Read the model definition and answer for the solid it produces. Units are mm, in the model's axes. A direction names the side the tool comes from. Coordinates: 2 decimals unless noted, no trailing zeros. Loops run counter-clockwise (first coordinate to the right, second up) from the corner with the lowest first, then second, coordinate; pieces in that order, holes last. Notation, with made-up numbers: (12.5, 65.5) - (49.5, 65.5) arc R30 cw to (49.5, 101.5) - close; hole circle Ø5 at (22, 7.25). An arc over 180 degrees is marked (long way). Use CSV: the item, a comma, the result in double quotes.
```python
from build123d import *

# Parameters (mm, degrees)
BOSS_EXTRUDE5_DEPTH = 3.175
SKETCH8_R           = 1.27
BOSS_EXTRUDE6_DEPTH = 3.302
CUT_EXTRUDE3_DEPTH  = 30.47138916


with BuildPart() as part:
    # Sketch7 → Boss-Extrude5 (new body)
    with BuildSketch(Plane(origin=(0, 0, 0), x_dir=(1, 0, 0), z_dir=(0, 1, 0))):
        with BuildLine():
            Line((-3.175, 25.4), (-3.175, -25.4))
            ThreePointArc((-3.175, -25.4), (0, -28.575), (3.175, -25.4))
            Line((3.175, -25.4), (3.175, 25.4))
            ThreePointArc((3.175, 25.4), (0, 28.575), (-3.175, 25.4))
        make_face()
    extrude(amount=BOSS_EXTRUDE5_DEPTH)

    # Sketch8 → Boss-Extrude6 (add)
    with BuildSketch(Plane(origin=(0, 3.175, 0), x_dir=(1, 0, 0), z_dir=(0, 1, 0))):
        with Locations(Location((0, 25.4, 0), (0, 0, 90))):
            Circle(SKETCH8_R)
        with Locations(Location((0, -25.4, 0), (0, 0, 90))):
            Circle(SKETCH8_R)
    extrude(amount=BOSS_EXTRUDE6_DEPTH)

    # Sketch9 → Cut-Extrude3 (cut, through all)
    with BuildSketch(Plane.XZ):
        with BuildLine():
            Line((-1.866511184, 1.905), (-1.866511184, -1.905))
            ThreePointArc((-1.866511184, -1.905), (0, -2.667), (1.866511184, -1.905))
            Line((1.866511184, -1.905), (1.866511184, 1.905))
            ThreePointArc((1.866511184, 1.905), (0, 2.667), (-1.866511184, 1.905))
        make_face()
    extrude(amount=-CUT_EXTRUDE3_DEPTH, mode=Mode.SUBTRACT)


solid = part.part
```
Q1. Given P1, Ø3, axis at x = 1.5, z = 1, coming from the +Y side (3 decimals), flat-ended and moving along its own axis, determine where the tip first touches the part or whether it passes through.
Reported:
P1,"stops at y = 3.175"
Q2. For a pull along Z with two mould halves and no side action, classify faces 1 (the face through (3.175, 2, 0)), 2 (the face through (-0.029, 1.565, -2.667)), 3 (the face through (0.07, 1.565, -28.574)) as +Z half, -Z half, draft (parallel to the pull), parting line (faces both ways), or undercut.
Reported:
face 1,"draft"
face 2,"undercut"
face 3,"-Z half"
Q3. A tool of negligible diameter and unlimited length cuts with its end or side. For faces 4 (the face through (-0.38, 4.8, -26.61)), 5 (the face through (0.029, 1.565, 2.667)), 6 (the face through (0, 6.477, -25)), from which of +Z, -Z, +X, -X, +Y, -Y can it reach the whole face along a straight path? Write none if from no direction.
Reported:
face 4,"+Y"
face 5,"+Y, -Y"
face 6,"+Z, -Z, +X, -X, +Y"
Q4. The part is cut by section B-B on y = 5. Determine the outline of the cut face in (x, z), and give its area (3 significant figures).
Reported:
outline,"circle Ø2.54 at (0, -25.4); circle Ø2.54 at (0, 25.4)"
area,"10.1 mm²"
Q5. The part is cut by section C-C on z = 7. Determine the outline of the cut face in (x, y) (3 decimals), and give its area (3 significant figures).
Reported:
outline,"(-3.175, 0) - (3.175, 0) - (3.175, 3.175) - (-3.175, 3.175) - close"
area,"20.2 mm²"
Q6. The part is cut by section A-A on x = 0. Determine the outline of the cut face in (y, z) (3 decimals), and give its area (3 significant figures).
Reported:
outline,"(0, -28.575) - (3.175, -28.575) - (3.175, -26.67) - (6.477, -26.67) - (6.477, -24.13) - (3.175, -24.13) - (3.175, -2.667) - (0, -2.667) - close; (0, 2.667) - (3.175, 2.667) - (3.175, 24.13) - (6.477, 24.13) - (6.477, 26.67) - (3.175, 26.67) - (3.175, 28.575) - (0, 28.575) - close"
area,"181 mm²"
Q7. Find the intervals of material crossed by probe 1 along Y at (x, z) = (-2.25, -8.5) (3 decimals); probe 2 along X at (y, z) = (1, 2) (3 decimals); probe 3 along Z at (x, y) = (1.5, 1.5), in increasing order. Write a range as [from, to].
Reported:
probe 1,"y = [0, 3.175]"
probe 2,"x = [-3.175, -1.764], [1.764, 3.175]"
probe 3,"z = [-28.2, -2.21], [2.21, 28.2]"
